Read the model definition and answer for the solid it produces. Units are mm, in the model's axes. Coordinates: 2 decimals unless noted, no trailing zeros. Order: outer loops, then holes, each group sorted by start corner. A loop starts at its lowest first (then second) coordinate and runs counter-clockwise, first axis right, second up.
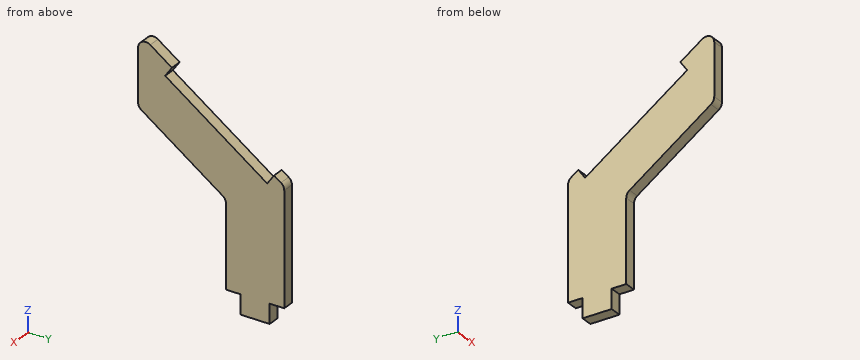
```python
from build123d import *

# Parameters (mm, degrees)
BOSS_EXTRUDE1_DEPTH = 3
CUT_EXTRUDE1_DEPTH  = 3


with BuildPart() as part:
    # Sketch2 → Boss-Extrude1 (new body)
    with BuildSketch(Plane(origin=(0, 0, 0), x_dir=(0, 0, -1), z_dir=(1, 0, 0))):
        with BuildLine():
            Line((0, -99.604434048), (-28.958865899, -99.604434048))
            ThreePointArc((-28.958865899, -99.604434048), (-29.882363125, -99.830412381), (-30.597169987, -100.457281175))
            Line((-30.597169987, -100.457281175), (-54.180855907, -134.138275212))
            ThreePointArc((-54.180855907, -134.138275212), (-54.316573485, -136.208925312), (-52.542551818, -137.285428085))
            Line((-52.542551818, -137.285428085), (-39.114031342, -137.285428085))
            ThreePointArc((-39.114031342, -137.285428085), (-38.190534115, -137.059449751), (-37.475727253, -136.432580958))
            Line((-37.475727253, -136.432580958), (-22.788664229, -115.457281175))
            ThreePointArc((-22.788664229, -115.457281175), (-22.073857367, -114.830412381), (-21.150360141, -114.604434048))
            Line((-21.150360141, -114.604434048), (0, -114.604434048))
            Line((0, -114.604434048), (0, -110.854434048))
            Line((0, -110.854434048), (5, -110.854434048))
            Line((5, -110.854434048), (5, -103.354434048))
            Line((5, -103.354434048), (0, -103.354434048))
            Line((0, -103.354434048), (0, -99.604434048))
        make_face()
    extrude(amount=BOSS_EXTRUDE1_DEPTH)

    # Sketch3 → Cut-Extrude1 (cut)
    with BuildSketch(Plane.ZY):
        Polygon((50.2661846, -128.547545189), (47.759579345, -130.302689084), (29.336304209, -103.991525421), (31.842909464, -102.236381526), align=None)
    extrude(amount=-CUT_EXTRUDE1_DEPTH, mode=Mode.SUBTRACT)


solid = part.part
```
1) A cutting plane is placed at C-C, the plane y = -110. Determine the outline of the cut face in (x, z), and give its area (3 significant figures).
A:
outline: (0, -5) - (3, -5) - (3, 33.54) - (0, 33.54) - close
area: 116 mm2
2) Straight lines are drawn through the part: line 1 (Y direction, x = 2.8, z = 4); line 2 (Z direction, x = 2.85, y = -104); line 3 (Y direction, x = 2.3, z = -1). For each, find the intervals that lie inside material, in ascending order.
A:
line 1: y = -114.6 to -99.6
line 2: z = -5 to 29.34
line 3: y = -110.85 to -103.35
3) A cutting plane is placed at A-A, the plane x = 1.45. Determine the outline of the cut face in (y, z).
A:
outline: (-137.29, 39.11) arc R2 ccw to (-136.43, 37.48) - (-115.46, 22.79) arc R2 cw to (-114.6, 21.15) - (-114.6, 0) - (-110.85, 0) - (-110.85, -5) - (-103.35, -5) - (-103.35, 0) - (-99.6, 0) - (-99.6, 28.96) arc R2 ccw to (-100.46, 30.6) - (-102.24, 31.84) - (-103.99, 29.34) - (-130.3, 47.76) - (-128.55, 50.27) - (-134.14, 54.18) arc R2 ccw to (-137.29, 52.54) - close
4) A cutting plane is placed at B-B, the plane z = 10.5. Determine the outline of the cut face in (x, y), and give its area (3 significant figures).
A:
outline: (0, -114.6) - (3, -114.6) - (3, -99.6) - (0, -99.6) - close
area: 45.0 mm2
5) Flat-ended cylindrical pins translate along their axes: pin 1 Ø1.5 at (x, z) = (1.5, -1.5) entering from +Y; pin 2 Ø1.5 at (x, z) = (2, 7.5) entering from -Y; pin 3 Ø1.5 at (x, y) = (1.5, -100.5) entering from -Z. Find the tip coordinate at first contact, or state that the pin passes through.
A:
pin 1: stops at y = -103.35
pin 2: stops at y = -114.6
pin 3: stops at z = 0
